Can you work these out from the model? Positions are in its coordinate system, mm. A direction names the side the tool comes from. Give positions to 0.01 mm unless a question says otherwise; leave off trailing zeros. Write each loop counter-clockwise with the first axis right and the second up, starting at its lowest first coordinate (ties: lowest second). Pieces come first, ordered by that corner, then holes. Notation, with made-up numbers: (-34.5, 14.25) -> (2.5, 14.25) arc R19 cw to (2.5, 23.25) -> close; hole circle Ø1 at (-15.75, -35.5). An arc over 180 degrees is marked (long way). One line per item, written item: value.
from build123d import *

# Parameters (mm, degrees)
SKETCH1_W           = 73.66656521
SKETCH1_H           = 1.5
BOSS_EXTRUDE1_DEPTH = 67.38
SKETCH2_R           = 2
BOSS_EXTRUDE2_DEPTH = 8
SKETCH3_R           = 0.9
CUT_EXTRUDE1_DEPTH  = 8
SKETCH4_R           = 2
BOSS_EXTRUDE3_DEPTH = 8
SKETCH5_R           = 0.9
CUT_EXTRUDE2_DEPTH  = 8


with BuildPart() as part:
    # Sketch1 → Boss-Extrude1 (new body)
    with BuildSketch(Plane.XY):
        with Locations((-252.623812979, 18.882492425)):
            Rectangle(SKETCH1_W, SKETCH1_H)
    extrude(amount=BOSS_EXTRUDE1_DEPTH)

    # Sketch2 → Boss-Extrude2 (add)
    with BuildSketch(Plane(origin=(0, 0, 0), x_dir=(-1, 0, 0), z_dir=(0, 0, -1))):
        with Locations((283.750452743, 17.632492425)):
            Circle(SKETCH2_R)
        with Locations((222.491552839, 17.632492425)):
            Circle(SKETCH2_R)
    extrude(amount=-BOSS_EXTRUDE2_DEPTH)

    # Sketch3 → Cut-Extrude1 (cut)
    with BuildSketch(Plane(origin=(0, 0, 0), x_dir=(-1, 0, 0), z_dir=(0, 0, -1))):
        with Locations((222.491552839, 17.632492425)):
            Circle(SKETCH3_R)
        with Locations((283.750452743, 17.632492425)):
            Circle(SKETCH3_R)
    extrude(amount=-CUT_EXTRUDE1_DEPTH, mode=Mode.SUBTRACT)

    # Sketch4 → Boss-Extrude3 (add)
    with BuildSketch(Plane.XY.offset(67.38)):
        with Locations((-222.491552839, 17.632492425)):
            Circle(SKETCH4_R)
        with Locations((-283.750452743, 17.632492425)):
            Circle(SKETCH4_R)
    extrude(amount=-BOSS_EXTRUDE3_DEPTH)

    # Sketch5 → Cut-Extrude2 (cut)
    with BuildSketch(Plane.XY.offset(67.38)):
        with Locations((-283.750452743, 17.632492425)):
            Circle(SKETCH5_R)
        with Locations((-222.491552839, 17.632492425)):
            Circle(SKETCH5_R)
    extrude(amount=-CUT_EXTRUDE2_DEPTH, mode=Mode.SUBTRACT)


solid = part.part
1) We'd pull the mould along Y, two halves only. Please class faces 4 (the face through (-284.46, 17.08, 63.44)), 5 (the face through (-215.791, 19, 33)), 6 (the face through (-253, 19.632, 33)): released by +Y, released by -Y, zero draft, split by the parting line, or undercut.
Answer list:
face 4: undercut
face 5: zero draft
face 6: released by +Y
2) If we section it at B-B (z = 38.5): Write out the boundary of the cut face in (x, y), and give its area (4 significant figures).
Answer list:
outline: (-289.46, 18.13) -> (-215.79, 18.13) -> (-215.79, 19.63) -> (-289.46, 19.63) -> close
area: 110.5 mm^2
3) If we section it at A-A (z = 4): Write out the boundary of the cut face in (x, y), and give its area (3 significant figures).
Answer list:
outline: (-289.46, 18.13) -> (-285.69, 18.13) arc R2 ccw (long way) to (-281.81, 18.13) -> (-224.43, 18.13) arc R2 ccw (long way) to (-220.56, 18.13) -> (-215.79, 18.13) -> (-215.79, 19.63) -> (-289.46, 19.63) -> close; hole circle Ø1.8 at (-283.75, 17.63); hole circle Ø1.8 at (-222.49, 17.63)
area: 122 mm^2
4) I need wall thicknesses on L1, parallel to X at y = 17.5, z = 3; L2, parallel to X at y = 18, z = 7; L3, parallel to Y at x = -276.5, z = 41.5. Which ranges of each line are inside material? Lowest first, please.
Answer list:
L1: x = -285.75 to -284.64, -282.86 to -281.75, -224.49 to -223.38, -221.6 to -220.5
L2: x = -285.72 to -284.57, -282.93 to -281.78, -224.46 to -223.31, -221.67 to -220.53
L3: y = 18.13 to 19.63
5) Will these pins go through, and if not, where does the flat tip stop? pin 1 (1 mm diameter, centred on y = 17.5, z = 8, fed in from -X); pin 2 (1.6 mm diameter, centred on x = -222.49, y = 17.63, fed in from -Z); pin 3 (1 mm diameter, centred on x = -231.5, y = 16.5, fed in from -Z); pin 4 (8 mm diameter, centred on x = -264.5, z = 22.5, fed in from -Y).
Answer list:
pin 1: stops at x = -285.75
pin 2: stops at z = 8
pin 3: passes through
pin 4: stops at y = 18.13
6) For faces 1 (the face through (-222.687, 16.754, 63.436)), 2 (the face through (-222, 16.6, 8)), 3 (the face through (-222.296, 16.754, 3.944)), which set-ups out of +Z, -Z, +X, -X, +Y, -Y let a thin tool reach every point of the face, with its end or its side?
Answer list:
face 1: +Z
face 2: +X, -X, -Y
face 3: -Z
7) If we section it at C-C (x = -273): Write out the boundary of the cut face in (y, z), and give its area (3 significant figures).
Answer list:
outline: (18.13, 0) -> (19.63, 0) -> (19.63, 67.38) -> (18.13, 67.38) -> close
area: 101 mm^2
